from build123d import *

# Parameters (mm, degrees)
BOSS_EXTRUDE1_DEPTH = 3
SKETCH12_R          = 2
CUT_EXTRUDE1_DEPTH  = 11


with BuildPart() as part:
    # Sketch11 → Boss-Extrude1 (new body)
    with BuildSketch(Plane(origin=(0, 0, 0), x_dir=(1, 0, 0), z_dir=(0, 1, 0))):
        with BuildLine():
            Line((-55.752395734, -4.879563459), (-55.752395734, -20.879563459))
            ThreePointArc((-55.752395734, -20.879563459), (-54.580822858, -23.707990583), (-51.752395734, -24.879563459))
            Line((-51.752395734, -24.879563459), (12.247604266, -24.879563459))
            ThreePointArc((12.247604266, -24.879563459), (15.076031391, -23.707990583), (16.247604266, -20.879563459))
            Line((16.247604266, -20.879563459), (16.247604266, -4.879563459))
            ThreePointArc((16.247604266, -4.879563459), (15.076031391, -2.051136334), (12.247604266, -0.879563459))
            Line((12.247604266, -0.879563459), (-51.752395734, -0.879563459))
            ThreePointArc((-51.752395734, -0.879563459), (-54.580822858, -2.051136334), (-55.752395734, -4.879563459))
        make_face()
    extrude(amount=BOSS_EXTRUDE1_DEPTH)

    # Sketch12 → Cut-Extrude1 (cut)
    with BuildSketch(Plane(origin=(0, 0, 0), x_dir=(1, 0, 0), z_dir=(0, 1, 0))):
        with Locations(Location((-51.752395734, -4.879563459, 0), (0, 0, 270))):
            Circle(SKETCH12_R)
        with Locations(Location((-43.752395734, -4.879563459, 0), (0, 0, 270))):
            Circle(SKETCH12_R)
        with Locations(Location((-35.752395734, -4.879563459, 0), (0, 0, 270))):
            Circle(SKETCH12_R)
        with Locations(Location((-27.752395734, -4.879563459, 0), (0, 0, 270))):
            Circle(SKETCH12_R)
        with Locations(Location((-19.75306076, -4.982713721, 0), (0, 0, 270))):
            Circle(SKETCH12_R)
        with Locations(Location((-11.75306076, -4.982713721, 0), (0, 0, 270))):
            Circle(SKETCH12_R)
        with Locations(Location((-3.75306076, -4.982713721, 0), (0, 0, 270))):
            Circle(SKETCH12_R)
        with Locations(Location((4.24693924, -4.982713721, 0), (0, 0, 270))):
            Circle(SKETCH12_R)
        with Locations(Location((12.247604266, -4.879563459, 0), (0, 0, 270))):
            Circle(SKETCH12_R)
        with Locations(Location((-51.752395734, -20.879563459, 0), (0, 0, 270))):
            Circle(SKETCH12_R)
        with Locations(Location((-43.752395734, -20.879563459, 0), (0, 0, 270))):
            Circle(SKETCH12_R)
        with Locations(Location((-35.752395734, -20.879563459, 0), (0, 0, 270))):
            Circle(SKETCH12_R)
        with Locations(Location((-27.752395734, -20.879563459, 0), (0, 0, 270))):
            Circle(SKETCH12_R)
        with Locations(Location((-19.752395734, -20.879563459, 0), (0, 0, 270))):
            Circle(SKETCH12_R)
        with Locations(Location((-11.752395734, -20.879563459, 0), (0, 0, 270))):
            Circle(SKETCH12_R)
        with Locations(Location((-3.752395734, -20.879563459, 0), (0, 0, 270))):
            Circle(SKETCH12_R)
        with Locations(Location((4.247604266, -20.879563459, 0), (0, 0, 270))):
            Circle(SKETCH12_R)
        with Locations(Location((12.247604266, -20.879563459, 0), (0, 0, 270))):
            Circle(SKETCH12_R)
        with BuildLine():
            Line((10.247604266, -14.982713721), (-49.752395734, -14.982713721))
            ThreePointArc((-49.752395734, -14.982713721), (-51.752395734, -12.982713721), (-49.752395734, -10.982713721))
            Line((-49.752395734, -10.982713721), (10.247604266, -10.982713721))
            ThreePointArc((10.247604266, -10.982713721), (12.247604266, -12.982713721), (10.247604266, -14.982713721))
        make_face()
    extrude(amount=CUT_EXTRUDE1_DEPTH, mode=Mode.SUBTRACT)


solid = part.part
CAD build for the part. Positions are in the model's coordinates, mm. A direction names the side the tool comes from. Coordinates: 2 decimals unless noted, no trailing zeros. Write each loop counter-clockwise with the first axis right and the second up, starting at its lowest first coordinate (ties: lowest second). Pieces come first, ordered by that corner, then holes. Notation, with made-up numbers: (64.5, 52) - (85.5, 52) arc R11 cw to (85.5, 68) - close; hole circle Ø3 at (-38.5, -39). An arc over 180 degrees is marked (long way). Use a Markdown table: item, result. Add a question column.
Item 1: Band-saw the part on A-A, the plane x = 9. Give the cut face in (y, z).
Item 2: Drill centre lines: L1, parallel to Z at x = -20, y = 0.75; L2, parallel to Z at x = -46, y = 1.1; L3, parallel to Z at x = 12, y = 2.25. Where is each one in solid material? Low to high. Write a range as from..to.
Item 3: Mould opens along X. For faces 3 (the face through (15.045, 1.479, 23.739)), 4 (the face through (-11.2, 1.5, 22.8)), 5 (the face through (-20, 1, 24.88)) say: pulls with the +X half, pulls with the -X half, needs draft (parallel to the pull), parting line crosses it, or undercut.
Item 4: Band-saw the part on C-C, the plane y = 0.8. Give the number of separate pieces and of enclosed holes in the cut face, and give its area (3 significant figures).
Item 5: Band-saw the part on B-B, the plane x = -10.5. Give the cut face in (y, z), and give its area (3 significant figures).
Item 6: Band-saw the part on D-D, the plane x = -44.5. Give the cut face in (y, z), and give its area (3 significant figures).
Item 7: 3-axis set-ups, long thin cutter, end or side, ignore diameter. For faces 1 (the face through (-20, 1, 10.983)), 2 (the face through (-54.55, 1.48, 2.02)): which of +Z, -Z, +X, -X, +Y, -Y reach the whole face in a straight line?
Numbers:
| question | item | result |
|---|---|---|
| 1 | outline | (0, 0.88) - (3, 0.88) - (3, 10.98) - (0, 10.98) - close; (0, 14.98) - (3, 14.98) - (3, 24.88) - (0, 24.88) - close |
| 2 | L1 | 0.88..3, 6.97..10.98, 14.98..18.89, 22.86..24.88 |
| 2 | L2 | 0.88..10.98, 14.98..24.88 |
| 2 | L3 | 0.88..2.89, 6.86..12.02, 13.95..18.89, 22.86..24.88 |
| 3 | face 3 | pulls with the +X half |
| 3 | face 4 | undercut |
| 3 | face 5 | needs draft |
| 4 | separate pieces | 1 |
| 4 | enclosed holes | 19 |
| 4 | area | 1,240 mm2 |
| 5 | outline | (0, 0.88) - (3, 0.88) - (3, 3.42) - (0, 3.42) - close; (0, 6.54) - (3, 6.54) - (3, 10.98) - (0, 10.98) - close; (0, 14.98) - (3, 14.98) - (3, 19.32) - (0, 19.32) - close; (0, 22.44) - (3, 22.44) - (3, 24.88) - (0, 24.88) - close |
| 5 | area | 41.3 mm2 |
| 6 | outline | (0, 0.88) - (3, 0.88) - (3, 3.02) - (0, 3.02) - close; (0, 6.73) - (3, 6.73) - (3, 10.98) - (0, 10.98) - close; (0, 14.98) - (3, 14.98) - (3, 19.02) - (0, 19.02) - close; (0, 22.73) - (3, 22.73) - (3, 24.88) - (0, 24.88) - close |
| 6 | area | 37.7 mm2 |
| 7 | face 1 | +Y, -Y |
| 7 | face 2 | -Z, -X, +Y, -Y |
